Can you work these out from the model? Positions are in its coordinate system, mm. A direction names the side the tool comes from. Give positions to 0.01 mm unless a question says otherwise; leave off trailing zeros. Order: outer loops, then holes, each group sorted by start corner. A loop starts at its lowest first (then second) coordinate and runs counter-clockwise, first axis right, second up. Notation, with made-up numbers: (55, -28) - (93, -28) arc R21 cw to (93, -17) - close; hole circle Ø11 at (-16.5, -11). An arc over 180 degrees is marked (long way). Use one line per item in the form item = value. Start each with the question number.
1) Suppose I cut it at B-B, the plane z = 38.25. Write out the boundary of the cut face in (x, y), and give its area (3 significant figures).
2) Which directions (+Z, -Z, +X, -X, +Y, -Y) give clear straight access to the entire face, cutting with the end or side of a thin tool? Please do faces 4 (the cylindrical face through (-28.89, -26.91, 31.58)), 5 (the flat face through (-37, -27, 46.581)).
3) We'd pull the mould along X, two halves only. Please class faces 1 (the cylindrical face through (-40.746, -13.928, 48.384)), 2 (the flat face through (-36, -8.23, 48)), 3 (the flat face through (-30.371, -28, 45)): released by +X, released by -X, zero draft, split by the parting line, or undercut.
4) For pin 1 (3 mm diameter, centred on y = -26, z = 34.5, fed in from +X); pin 2 (6 mm diameter, centred on x = -30.5, y = -36, fed in from -Z); pin 3 (2 mm diameter, centred on x = -29.5, z = 34, fed in from -Y); pin 4 (4 mm diameter, centred on x = -30, z = 37, fed in from -Y), each with a flat end and sliding along its axis, tell me the tip position at first contact or that it passes through.
5) Suppose I cut it at C-C, the plane x = -35.75. Write out the boundary of the cut face in (y, z).
6) Suppose I cut it at D-D, the plane x = -40. State how many separate pieces and enclosed holes the cut face has, and give its area (3 significant figures).
7) Suppose I cut it at A-A, the plane y = -24. Write out the boundary of the cut face in (x, z).
8) Please list where these lines run through material, in increasing order: probe 1 along Z at (x, y) = (-29, -27); probe 2 along Z at (x, y) = (-36, -44); probe 3 along Z at (x, y) = (-27.75, -31).
Autodesk Inventor part; units mm, degrees
ref_plane "YZ Plane" through (0, 0, 0) normal (1, 0, 0) x (0, 1, 0)
ref_plane "XZ Plane" through (0, 0, 0) normal (0, 1, 0) x (-1, 0, 0)
ref_plane "XY Plane" through (0, 0, 0) normal (0, 0, 1) x (1, 0, 0)
ref_plane "Work Plane1" through (-14.6708, -27.7298, 48.581) normal (0, 0, -1) x (-1, 0, 0)
sketch "Sketch1" plane through (-14.6708, -27.7298, 48.581) normal (0, 0, -1) x (-1, 0, 0)
  circle A0 centre (26, 15.5) radius 3.3
  circle A1 centre (26, -14) radius 3.3
  line L0 (12.7, 19.5) -> (30, 19.5)
  line L1 (30, 19.5) -> (30, -18)
  line L2 (30, -18) -> (12.7, -18)
  line L3 (12.7, -18) -> (12.7, 19.5)
  line L4 (15.7, 19.5) -> (15.7, -18)
  point P0 (-14.6708, 27.7298)
  dimension "d0" = 4
  dimension "d1" = 4
  dimension "d2" = 4
  dimension "d3" = 10
  dimension "d4" = 3
extrude "Extrusion1" add sketch "Sketch1" along normal blind 2 contours A0 | A1 | L0 L4 L2 L3 | L0 L1 L2 L4
sketch "Sketch2" plane through (-14.6708, -27.7298, 46.581) normal (0, 0, -1) x (-1, 0, 0)
  line L0 (15.7, 19.5) -> (15.7, -18)
  line L1 (12.7, 19.5) -> (12.7, -18)
  circle A0 centre (26, 15.5) radius 3.3
  circle A1 centre (26, -14) radius 3.3
  line L2 (30, 19.5) -> (12.7, 19.5)
  line L3 (12.7, -18) -> (30, -18)
  point P0 (-14.6708, 27.7298)
hole "Hole1" at (-40.6708, -12.2298, 46.581) at (-40.6708, -41.7298, 46.581) direction (0, 0, 1) diameter 3.4 end through all countersink diameter 6.6 countersink angle 90
sketch "Sketch3" plane through (-14.6708, -27.7298, 46.581) normal (0, 0, -1) x (-1, 0, 0)
  line L0 (30, 19.5) -> (12.7, 19.5)
  line L1 (12.7, 19.5) -> (12.7, -18)
  line L2 (15.7, 19.5) -> (15.7, -18)
  line L3 (12.7, -18) -> (30, -18)
  point P0 (-14.6708, 27.7298)
extrude "Extrusion2" add sketch "Sketch3" along normal blind 62.25
sketch "Sketch4" plane through (-30.3708, -45.7298, 46.581) normal (-1, 0, 0) x (0, 0, 1)
  line L0 (2, 0) -> (-62.25, 0)
  line L1 (-8, 0) -> (-8, 37.5) construction
  line L2 (0, 37.5) -> (-62.25, 37.5)
  circle A0 centre (-8, 18.75) radius 7
  line L3 (0, 37.5) -> (0, 0)
  circle A1 centre (-8, 18.75) radius 6
  line L4 (0, 0) -> (-13.1037, 13.9591)
  line L5 (-13.1037, 23.5409) -> (0, 37.5)
  line L6 (-62.25, 0) -> (-62.25, 37.5)
  point P0 (-46.581, 45.7298)
  dimension "d16" = 14
  dimension "d17" = 8
  dimension "d18" = 12
extrude "Extrusion3" cut sketch "Sketch4" against normal through all contours L0 L6 L2 L5 A0 L4 | A1
properties part number "tumbler_holder"
Result sheet:
q1.outline = (-30.37, -36.85) - (-27.37, -36.85) - (-27.37, -32.97) - (-30.37, -32.97) - close; (-30.37, -20.99) - (-27.37, -20.99) - (-27.37, -17.1) - (-30.37, -17.1) - close
q1.area = 23.3 mm²
q2.face_4 = -Z, +X, -X
q2.face_5 = -Z, -X, +Y, -Y
q3.face_1 = undercut
q3.face_2 = zero draft
q3.face_3 = released by -X
q4.pin_1 = through
q4.pin_2 = 34.63
q4.pin_3 = -33.39
q4.pin_4 = -37.65
q5.outline = (-45.73, 46.58) - (-8.23, 46.58) - (-8.23, 48.58) - (-45.73, 48.58) - close
q6.separate_pieces = 3
q6.enclosed_holes = 0
q6.area = 57.1 mm²
q7.outline = (-44.67, 46.58) - (-30.37, 46.58) - (-30.37, 43.79) - (-27.37, 43.79) - (-27.37, 48.58) - (-44.67, 48.58) - close; (-30.37, 32.25) - (-27.37, 32.25) - (-27.37, 33.37) - (-30.37, 33.37) - close
q8.probe_1 = 31.58 to 32.58, 44.58 to 48.58
q8.probe_2 = 46.58 to 48.58
q8.probe_3 = 32.85 to 34.13, 43.03 to 48.58
